Model file for the job. Use its own axes, mm. A direction names the side the tool comes from. Coordinates: 2 decimals unless noted, no trailing zeros. Write each loop counter-clockwise with the first axis right and the second up, starting at its lowest first coordinate (ties: lowest second). Pieces come first, ordered by that corner, then holes. Notation, with made-up numbers: M -4.5,31 L 32.5,31 A28 cw 32.5,50 Z; hole C -25.5,4.25 d9. An arc over 180 degrees is marked long. One line per question, with ' | ' between items. Start each with the question number.
(1) Cut at D-D (z = 26). Write the cut outline in (x, y).
(2) Flat gauge pins, fed straight in: pin 1 Ø10 at (x, y) = (-6, -19.5) entering from -Z; pin 2 Ø24 at (y, z) = (-9.5, 43.5) entering from +X; pin 3 Ø3 at (x, y) = (49, -38) entering from +Z. Where does each tip first touch, or does it go through?
(3) Cut at C-C (x = 38.5). Write the cut outline in (y, z).
(4) Cut at A-A (y = 2). Write the cut outline in (x, z).
(5) Two-plate mould, pull along Y, no slides. Class faces 6 (the face through (62, 61.214, 37)), 7 (the face through (-5, -61, 177.8)), 8 (the face through (2, 63.5, 103)): +Y half, -Y half, draft (parallel to the pull), parting line (faces both ways), or undercut.
(6) Wall check: probe 1 along Y at (x, z) = (21, 78.5); probe 2 along Z at (x, y) = (43, -3). Give the ranges that are in metal, low to high.
(7) Cut at B-B (z = 168.5). Write the cut outline in (x, y).
(8) Tool access for faces 1 (the face through (2, -63.5, 103)), 2 (the face through (-63.5, -1, 121)), 3 (the face through (-1.374, -0.889, 37.755)), 4 (the face through (-1, -59.69, 113)), 5 (the face through (62, -61.214, 37)): list every direction of +Z, -Z, +X, -X, +Y, -Y with a clear straight run to the whole face (end or side of a thin tool).
from build123d import *

# Parameters (mm, degrees)
F0_W      = 127
F0_H      = 127
F0_W_2    = 119.38
F0_H_2    = 119.38
F1_DEPTH  = 177.8
F10_DEPTH = 127.001
F11_W     = 137.4053613401
F11_H     = 127
F12_DEPTH = 1.27
F13_W     = 122.4279999733
F13_H     = 48.0059999866
F14_DEPTH = 3.81


# Not quite as in the source:
# - a feature of the source that left no trace in its solid (it failed there, or was rolled back) is left out
# - a feature names something its author has since deleted; it is built from what else it names


with BuildPart() as f1:
    # F0 (on Top) → F1 (new body)
    with BuildSketch(Plane.XY):
        Rectangle(F0_W, F0_H)
        Rectangle(F0_W_2, F0_H_2, mode=Mode.SUBTRACT)
    extrude(amount=F1_DEPTH)

    # F8: union 

    # F9 (on face) → F10 (cut, through all)
    with BuildSketch(Plane.XZ.offset(63.5)):
        Polygon((75.6702050567, -13.2453246042), (93.3672711253, 0), (-89.8822396994, 75.6837800145), (-89.8822396994, -21.479823067), align=None)
    extrude(amount=-F10_DEPTH, mode=Mode.SUBTRACT)

    # F11 (on face) → F12 (join)
    with BuildSketch(Plane(origin=(13.6055070593, 0, 32.9423624542), x_dir=(0.924272523, 0, -0.3817332881), z_dir=(-0.3817332881, 0, -0.924272523))):
        with Locations((-14.7202331787, 0)):
            Rectangle(F11_W, F11_H)
    extrude(amount=F12_DEPTH)

    # F13 (on face) → F14 (cut)
    with BuildSketch(Plane.YZ.offset(63.5)):
        with Locations((0, 36.8464652686)):
            Rectangle(F13_W, F13_H)
    extrude(amount=-F14_DEPTH, mode=Mode.SUBTRACT)


solid = f1.part
Filled in:
1) outline: M 27.09,-63.5 L 63.5,-63.5 L 63.5,-61.21 L 59.69,-61.21 L 59.69,-59.69 L 30.41,-59.69 L 30.41,59.69 L 59.69,59.69 L 59.69,61.21 L 63.5,61.21 L 63.5,63.5 L 27.09,63.5 Z
2) pin 1: z = 37.6 | pin 2: x = 17.1 | pin 3: z = 18.94
3) outline: M -63.5,21.29 L 63.5,21.29 L 63.5,177.8 L 59.69,177.8 L 59.69,22.66 L -59.69,22.66 L -59.69,177.8 L -63.5,177.8 Z
4) outline: M -63.98,63.61 L 63.02,11.16 L 63.5,12.34 L 63.5,12.84 L 59.69,12.84 L 59.69,13.91 L -59.69,63.21 L -59.69,177.8 L -63.5,177.8 L -63.5,64.79 Z; M 59.69,60.85 L 63.5,60.85 L 63.5,177.8 L 59.69,177.8 Z
5) face 6: undercut | face 7: draft | face 8: +Y half
6) probe 1: -63.5 to -59.69, 59.69 to 63.5 | probe 2: 19.43 to 20.8
7) outline: M -63.5,-63.5 L 63.5,-63.5 L 63.5,63.5 L -63.5,63.5 Z; hole M -59.69,-59.69 L 59.69,-59.69 L 59.69,59.69 L -59.69,59.69 Z
8) face 1: +Z, -Z, +X, -X, -Y | face 2: +Z, -X, +Y, -Y | face 3: -Z, -X, +Y, -Y | face 4: +Z | face 5: +X
